Input: part model. Units: mm. Frame: model coordinates. Coordinates: 2 decimals unless noted, no trailing zeros. Loops run counter-clockwise (first coordinate to the right, second up) from the corner with the lowest first, then second, coordinate; pieces in that order, holes last.
Item 1: Section A-A on y = 311. Return loops of the section in (x, z).
Item 2: Ray query, line 1 along Z through (x, y) = (12.25, 942.5); line 2 along Z through (x, y) = (0.65, 26.75); line 3 along X through (y, z) = (540, -8.25). Return the intervals inside material, ascending.
Item 3: Contact query for a flat-ended pin moving along its axis: P1, Ø1.5, axis at y = 747, z = -6, coming from the -X side. Output: stop coordinate, or through.
Autodesk Inventor part; units mm, degrees
ref_plane "YZ Plane" through (0, 0, 0) normal (1, 0, 0) x (0, 1, 0)
ref_plane "XZ Plane" through (0, 0, 0) normal (0, 1, 0) x (-1, 0, 0)
ref_plane "XY Plane" through (0, 0, 0) normal (0, 0, 1) x (1, 0, 0)
sketch "スケッチ1" plane through (0, 0, 0) normal (0, 1, 0) x (-1, 0, 0)
  line L0 (0, 0) -> (-15, 0)
  line L1 (-15, 0) -> (-15, -15)
  line L2 (-15, -15) -> (0, -15)
  line L3 (0, -15) -> (0, 0)
  line L4 (-1.5, -1.5) -> (-13.5, -1.5)
  line L5 (-13.5, -1.5) -> (-13.5, -13.5)
  line L6 (-13.5, -13.5) -> (-1.5, -13.5)
  line L7 (-1.5, -13.5) -> (-1.5, -1.5)
  dimension "d0" = 15
  dimension "d1" = 15
  dimension "d2" = 12
  dimension "d3" = 12
  dimension "d4" = 1.5
  dimension "d5" = 1.5
extrude "押し出し1" add sketch "スケッチ1" along normal blind 1200
sketch "スケッチ3" plane through (15, 0, 0) normal (0, 0, 1) x (1, 0, 0)
  line L0 (-15, 0) -> (-15, 1200)
  line L1 (-15, 0) -> (0, 0)
  point P0 (-7.5, 7.5)
  point P1 (-7.5, 107.5)
  dimension "d8" = 7.5
  dimension "d9" = 7.5
  dimension "d10" = 7.5
  dimension "d11" = 100
hole "穴1" at (7.5, 7.5, 0) at (7.5, 107.5, 0) direction (0, 0, -1) diameter 3 end through all
sketch "スケッチ4" plane through (0, 0, 0) normal (-1, 0, 0) x (0, 0, 1)
  line L0 (-15, 0) -> (0, 0)
  line L1 (-15, 0) -> (-15, 1200)
  point P0 (-7.5, 16.5)
  point P1 (-7.5, 98.5)
  dimension "d19" = 16.5
  dimension "d20" = 7.5
  dimension "d21" = 7.5
  dimension "d22" = 82
hole "穴2" at (0, 16.5, -7.5) at (0, 98.5, -7.5) direction (1, 0, 0) diameter 3 end through all
sketch "スケッチ5" plane through (15, 0, -15) normal (1, 0, 0) x (0, 0, -1)
  line L0 (0, 0) -> (0, 1200)
  line L1 (-15, 1200) -> (0, 1200)
  point P0 (-15, 0)
  point P1 (-7.5, 1192.5)
  dimension "d30" = 7.5
  dimension "d31" = 7.5
hole "穴3" at (15, 1192.5, -7.5) direction (-1, 0, 0) diameter 3 end through all
sketch "スケッチ6" plane through (15, 0, 0) normal (0, 0, 1) x (1, 0, 0)
  circle A0 centre (-7.5, 7.5) radius 1.5
  circle A1 centre (-7.5, 107.5) radius 1.5
  line L0 (-7.5, 7.5) -> (-7.5, 107.5)
  point P0 (-15, 0)
  point P1 (-7.5, 17.5)
  point P2 (-7.5, 27.5)
  point P3 (-7.5, 37.5)
  point P4 (-7.5, 47.5)
  point P5 (-7.5, 57.5)
  point P6 (-7.5, 67.5)
  point P7 (-7.5, 77.5)
  point P8 (-7.5, 87.5)
  point P9 (-7.5, 97.5)
  dimension "d39" = 100
  dimension "d40" = 10
  dimension "d43" = 10
hole "穴4" at (7.5, 17.5, 0) at (7.5, 27.5, 0) at (7.5, 37.5, 0) at (7.5, 47.5, 0) at (7.5, 57.5, 0) at (7.5, 67.5, 0) at (7.5, 77.5, 0) at (7.5, 87.5, 0) at (7.5, 97.5, 0) direction (0, 0, -1) diameter 9 end through all
sketch "スケッチ7" plane through (15, 0, -15) normal (1, 0, 0) x (0, 0, -1)
  circle A0 centre (-7.5, 16.5) radius 1.5
  circle A1 centre (-7.5, 98.5) radius 1.5
  line L0 (-7.5, 16.5) -> (-7.5, 98.5)
  point P0 (-15, 0)
  point P1 (-7.5, 26.75)
  point P2 (-7.5, 37)
  point P3 (-7.5, 47.25)
  point P4 (-7.5, 57.5)
  point P5 (-7.5, 67.75)
  point P6 (-7.5, 78)
  point P7 (-7.5, 88.25)
  dimension "d55" = 82
  dimension "d56" = 10.25
  dimension "d59" = 10.25
hole "穴5" at (15, 26.75, -7.5) at (15, 37, -7.5) at (15, 47.25, -7.5) at (15, 57.5, -7.5) at (15, 67.75, -7.5) at (15, 78, -7.5) at (15, 88.25, -7.5) direction (-1, 0, 0) diameter 9 end through all
sketch "スケッチ8" plane through (15, 0, -15) normal (1, 0, 0) x (0, 0, -1)
  line L0 (-15, 0) -> (-15, 1200)
  line L1 (-15, 0) -> (0, 0)
  circle A0 centre (-7.5, 98.5) radius 1.5
  point P0 (-7.5, 7.5)
  point P1 (-7.5, 107.5)
  dimension "d71" = 7.5
  dimension "d72" = 7.5
  dimension "d73" = 7.5
  dimension "d74" = 9
hole "穴6" at (15, 7.5, -7.5) at (15, 107.5, -7.5) direction (-1, 0, 0) diameter 9 end through all
equation "\"d3\" = d2"
equation "\"d4\" = d5"
properties part number "12ｘ12_1" material "アルミニウム 6061"
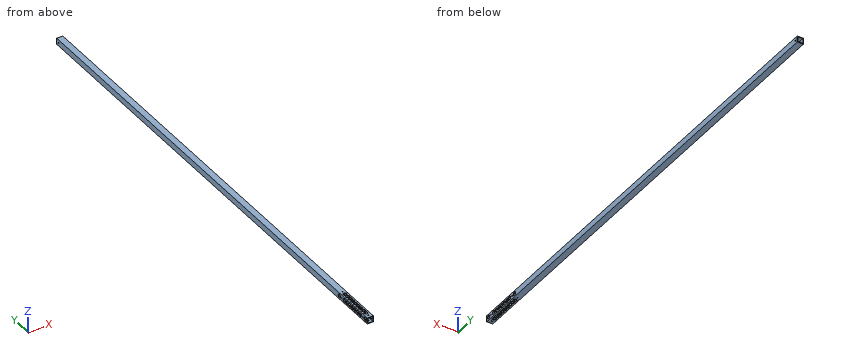
Results found:
1. outline: (0, -15) - (15, -15) - (15, 0) - (0, 0) - close; hole (1.5, -13.5) - (13.5, -13.5) - (13.5, -1.5) - (1.5, -1.5) - close
2. line 1: z = -15 to -13.5, -1.5 to 0
2. line 2: z = -15 to -12, -3 to 0
2. line 3: x = 0 to 1.5, 13.5 to 15
3. P1: stops at x = 0
